```python
from build123d import *

# Parameters (mm, degrees)
SKETCH1_R           = 19.05
BOSS_EXTRUDE1_DEPTH = 1.5875
FILLET1_R           = 6.35
SKETCH4_R           = 1.9939
BOSS_EXTRUDE2_DEPTH = 3.175


with BuildPart() as part:
    # Sketch1 → Boss-Extrude1 (new, symmetric)
    with BuildSketch(Plane(origin=(0, 0, 0), x_dir=(1, 0, 0), z_dir=(0, 1, 0))):
        with BuildLine():
            Line((0, 25.8572), (-22.49266633, 20.776091776))
            ThreePointArc((-22.49266633, 20.776091776), (-23.925232015, 19.108880164), (-25.234496658, 17.343189053))
            Line((-25.234496658, 17.343189053), (-25.258396026, 1.987878879))
            ThreePointArc((-25.258396026, 1.987878879), (-25.334329361, 0.331644538), (-25.301777207, -1.326009955))
            Line((-25.301777207, -1.326009955), (-21.651397508, -21.651397508))
            ThreePointArc((-21.651397508, -21.651397508), (-20.188971055, -23.021109353), (-18.640092328, -24.292241274))
            Line((-18.640092328, -24.292241274), (-3.375041857, -25.63598807))
            ThreePointArc((-3.375041857, -25.63598807), (-1.691141793, -25.80183775), (0, -25.8572))
            Line((0, -25.8572), (22.49266633, -20.776091776))
            ThreePointArc((22.49266633, -20.776091776), (23.925232015, -19.108880164), (25.234496658, -17.343189053))
            Line((25.234496658, -17.343189053), (25.258396026, -1.987878879))
            ThreePointArc((25.258396026, -1.987878879), (25.334329361, -0.331644538), (25.301777207, 1.326009955))
            Line((25.301777207, 1.326009955), (21.651397508, 21.651397508))
            ThreePointArc((21.651397508, 21.651397508), (20.188971055, 23.021109353), (18.640092328, 24.292241274))
            Line((18.640092328, 24.292241274), (3.375041857, 25.63598807))
            ThreePointArc((3.375041857, 25.63598807), (1.691141793, 25.80183775), (0, 25.8572))
        make_face()
        with Locations(Location((0, 0, 0), (0, 0, 270))):
            Circle(SKETCH1_R, mode=Mode.SUBTRACT)
    extrude(amount=BOSS_EXTRUDE1_DEPTH, both=True)

    # Fillet1
    # the kernel refuses this fillet: 6.35 mm, written as the material it takes off along each edge
    with BuildSketch(Plane(origin=(25.301777207, -2.821548673, -1.326009955), x_dir=(-0.17676882960283344, 0, -0.9842523969393442), z_dir=(0, 1, 0)), Plane(origin=(-25.301777207, -2.821548673, 1.326009955), x_dir=(0.17676882960285092, 0, 0.9842523969393412), z_dir=(0, 1, 0))) as fillet1_piece_1:
        with BuildLine():
            CenterArc((0.427308397, 6.35), FILLET1_R, 261.702105294, 8.297894706)
            ThreePointArc((-0.489122596, 0.066477562), (-0.244723196, 0.032047583), (0, 0))
            Line((0, 0), (0.427308397, 0))
        make_face()
    extrude(amount=5.643097347, mode=Mode.SUBTRACT)
    with BuildSketch(Plane(origin=(0, -3.771668691, -25.8572), x_dir=(0.9998572847598118, 0, 0.016894085140560105), z_dir=(0, 1, 0))) as fillet1_piece_2:
        with BuildLine():
            CenterArc((0.766390036, -6.349093758), FILLET1_R, 89.031994173, 14.665503243)
            Line((-0.737262724, -0.179691163), (0, 0))
            ThreePointArc((0, 0), (0.436833738, 0.003690217), (0.873667477, 0))
        make_face()
    extrude(amount=7.543337383, mode=Mode.SUBTRACT)
    with BuildSketch(Plane(origin=(-22.49266633, -7.488620609, -20.776091776), x_dir=(-0.649702048384586, 0, 0.7601889556714653), z_dir=(0, 1, 0)), Plane(origin=(22.49266633, -7.488620609, 20.776091776), x_dir=(0.6497020483845872, 0, -0.7601889556714644), z_dir=(0, 1, 0))) as fillet1_piece_3:
        with BuildLine():
            CenterArc((2.115690027, 6.345281193), FILLET1_R, 233.248632952, 38.960357221)
            Line((-1.683792582, 1.257410134), (0, 0))
            ThreePointArc((0, 0), (1.180224122, -0.022754088), (2.360448244, 0))
        make_face()
    extrude(amount=14.977241219, mode=Mode.SUBTRACT)
    with BuildSketch(Plane(origin=(-25.234496658, -7.46444532, -17.343189053), x_dir=(-0.0015564217956219107, 0, 0.9999987887748636), z_dir=(0, 1, 0)), Plane(origin=(25.234496658, -7.46444532, 17.343189053), x_dir=(0.0015564217956202159, 0, -0.9999987887748636), z_dir=(0, 1, 0))) as fillet1_piece_4:
        with BuildLine():
            CenterArc((2.092875431, 6.35), FILLET1_R, 231.189304273, 38.810695727)
            ThreePointArc((-1.886982522, 1.401946779), (-0.956950246, 0.682857958), (0, 0))
            Line((0, 0), (2.092875431, 0))
        make_face()
    extrude(amount=14.928890641, mode=Mode.SUBTRACT)
    with BuildSketch(Plane(origin=(-21.651397508, -7.539410962, 21.651397508), x_dir=(0.7340619600556395, 0, 0.6790824977860002), z_dir=(0, 1, 0))) as fillet1_piece_5:
        with BuildLine():
            CenterArc((2.133899558, 6.345199584), FILLET1_R, 232.953597243, 39.274415035)
            Line((-1.691731763, 1.276960738), (0, 0))
            ThreePointArc((0, 0), (1.190382192, -0.023147607), (2.380764385, 0))
        make_face()
    extrude(amount=15.078821924, mode=Mode.SUBTRACT)
    with BuildSketch(Plane(origin=(-18.640092328, -7.110021665, 24.292241274), x_dir=(0.9961479372781339, 0, 0.08768857996637193), z_dir=(0, 1, 0))) as fillet1_piece_6:
        with BuildLine():
            CenterArc((1.966659426, 6.35), FILLET1_R, 233.396238517, 36.603761483)
            ThreePointArc((-1.8197032, 1.252357597), (-0.92114894, 0.609763515), (0, 0))
            Line((0, 0), (1.966659426, 0))
        make_face()
    extrude(amount=14.22004333, mode=Mode.SUBTRACT)
    with BuildSketch(Plane(origin=(0, -3.771668691, 25.8572), x_dir=(0.9754212543155903, 0, -0.22034830752560894), z_dir=(0, 1, 0))) as fillet1_piece_7:
        with BuildLine():
            CenterArc((0.758844673, 6.35), FILLET1_R, 255.334496757, 14.665503243)
            ThreePointArc((-0.848819905, 0.206880711), (-0.42528378, 0.099855091), (0, 0))
            Line((0, 0), (0.758844673, 0))
        make_face()
    extrude(amount=7.543337383, mode=Mode.SUBTRACT)
    with BuildSketch(Plane(origin=(18.640092328, 7.110021665, -24.292241274), x_dir=(-0.9961479372781336, 0, -0.08768857996637594), z_dir=(0, -1, 0))) as fillet1_piece_8:
        with BuildLine():
            CenterArc((1.966659426, -6.35), FILLET1_R, 90, 36.603761483)
            ThreePointArc((-1.8197032, -1.252357597), (-0.92114894, -0.609763515), (0, 0))
            Line((0, 0), (1.966659426, 0))
        make_face()
    extrude(amount=14.22004333, mode=Mode.SUBTRACT)
    with BuildSketch(Plane(origin=(21.651397508, 7.539410962, -21.651397508), x_dir=(-0.7340619600556043, 0, -0.679082497786038), z_dir=(0, -1, 0))) as fillet1_piece_9:
        with BuildLine():
            CenterArc((2.133899558, -6.345199584), FILLET1_R, 87.771987722, 39.274415035)
            Line((-1.691731763, -1.276960738), (0, 0))
            ThreePointArc((0, 0), (1.190382192, 0.023147607), (2.380764385, 0))
        make_face()
    extrude(amount=15.078821924, mode=Mode.SUBTRACT)

    # Sketch4 → Boss-Extrude2 (add)
    with BuildSketch(Plane(origin=(0, 1.5875, 0), x_dir=(1, 0, 0), z_dir=(0, 1, 0))):
        with BuildLine():
            Line((18.171090284, -26.981546007), (20.442833543, -21.23915036))
            Line((20.442833543, -21.23915036), (16.989846709, -22.019182373))
            Line((16.989846709, -22.019182373), (11.9001109, -23.168957064))
            Line((11.9001109, -23.168957064), (3.07364609, -25.162861312))
            Line((3.07364609, -25.162861312), (10.75965287, -27.467658849))
            Line((10.75965287, -27.467658849), (10.523541405, -34.452658849))
            ThreePointArc((10.523541405, -34.452658849), (15.772035547, -39.203698132), (19.584588194, -33.238506824))
            Line((19.584588194, -33.238506824), (19.305744856, -32.004144185))
            Line((19.305744856, -32.004144185), (16.179043161, -29.213406378))
            Line((16.179043161, -29.213406378), (18.171090284, -26.981546007))
        make_face()
        with Locations(Location((15.156395368, -34.609261559, 0), (0, 0, 270))):
            Circle(SKETCH4_R, mode=Mode.SUBTRACT)
    extrude(amount=-BOSS_EXTRUDE2_DEPTH)


solid = part.part
```
Verification items for the finished model (mm, model axes). A direction names the side the tool comes from. Give positions to 0.01 mm unless a question says otherwise; leave off trailing zeros. Order: outer loops, then holes, each group sorted by start corner. A loop starts at its lowest first (then second) coordinate and runs counter-clockwise, first axis right, second up. Notation, with made-up numbers: (76, 40) -> (117, 40) arc R20 cw to (117, 62) -> close; hole circle Ø2 at (30.25, -17.75). An arc over 180 degrees is marked (long way). Use a Markdown table: item, result.
1) Depth check by flat-ended pin: pin 1 Ø6 at (x, z) = (-9, -10.5) entering from -Y; pin 2 Ø1.5 at (y, z) = (-1.5, -11.5) entering from +X. Enter the tip coordinate at first touch or a pass-through.
Results:
| item | result |
|---|---|
| pin 1 | through |
| pin 2 | x = 23.61 |
2) Section check A-A, the plane z = 0. Record the boundary of the cut face in (x, y), then the cut area to 3 significant figures.
Results:
| item | result |
|---|---|
| outline | (-25.34, -1.59) -> (-19.05, -1.59) -> (-19.05, 1.59) -> (-25.34, 1.59) -> close; (19.05, -1.59) -> (25.34, -1.59) -> (25.34, 1.59) -> (19.05, 1.59) -> close |
| area | 39.9 mm² |
3) Section check B-B, the plane x = 5.5. Record the boundary of the cut face in (y, z).
Results:
| item | result |
|---|---|
| outline | (-1.59, -25.45) -> (1.59, -25.45) -> (1.59, -18.24) -> (-1.59, -18.24) -> close; (-1.59, 18.24) -> (1.59, 18.24) -> (1.59, 25.89) -> (-1.59, 25.89) -> close |
4) Section check C-C, the plane z = 28.5. Record the boundary of the cut face in (x, y), then the cut area to 3 significant figures.
Results:
| item | result |
|---|---|
| outline | (10.72, -1.59) -> (16.82, -1.59) -> (16.82, 1.59) -> (10.72, 1.59) -> close |
| area | 19.3 mm² |
5) Tool access check on faces 1 (the cylindrical face through (-24.89, -0.02, -17.31)), 2 (the flat face through (17.764, 0.022, 30.628)), 3 (the cylindrical face through (-0.07, -0.02, 25.82)). Record the directions out of +Z, -Z, +X, -X, +Y, -Y that give a thin tool (end or side, any length) a straight path to the whole face; none if there is none.
Results:
| item | result |
|---|---|
| face 1 | -Z, -X, +Y, -Y |
| face 2 | +X, +Y, -Y |
| face 3 | +Z, +Y, -Y |
6) Mould release check, pull along Z, two halves, no side actions. Record for faces 4 (the cylindrical face through (-11.59, -0.02, -15.12)), 5 (the cylindrical face through (0.07, -0.02, -25.82)), 6 (the flat face through (1.89, 0.02, 25.43)), 7 (the cylindrical face through (16.84, 0.02, 35.68)): pulls with the +Z half, pulls with the -Z half, needs draft (parallel to the pull), parting line crosses it, or undercut.
Results:
| item | result |
|---|---|
| face 4 | undercut |
| face 5 | pulls with the -Z half |
| face 6 | pulls with the +Z half |
| face 7 | undercut |
7) Material ranges on probe 1 along X at (y, z) = (0, 0); probe 2 along Z at (x, y) = (14.5, -1); probe 3 along Z at (x, y) = (16, -0.05), recorded low to high.
Results:
| item | result |
|---|---|
| probe 1 | -25.34 to -19.05, 19.05 to 25.34 |
| probe 2 | -24.66 to -12.36, 12.36 to 32.73, 36.49 to 39.2 |
| probe 3 | -24.52 to -10.34, 10.34 to 32.8, 36.42 to 39.17 |
